Part model, mm, in its own coordinate system. Face numbers are marked on the shaded views. A direction names the side the tool comes from. Coordinates: 2 decimals unless noted, no trailing zeros. Write each loop counter-clockwise with the first axis right and the second up, starting at its lowest first coordinate (ties: lowest second). Pieces come first, ordered by that corner, then holes. Notation, with made-up numbers: (-12.5, -31.5) -> (19.5, -31.5) arc R24 cw to (19.5, -8.5) -> close; hole circle Ø6 at (-4.5, 76.25). An arc over 180 degrees is marked (long way). Write item = value, one per line. Start each with the question number.
Q1. Band-saw the part on C-C, the plane x = 29.5. List the corners of the cut face in (y, z).
Q2. Band-saw the part on D-D, the plane y = 8. List the corners of the cut face in (x, z).
Q3. Band-saw the part on A-A, the plane z = 28. List the corners of the cut face in (x, y).
Q4. Probe line 1 (Y direction, x = 29.5, z = 1.9); line 2 (Z direction, x = 1.65, y = 8); line 3 (Y direction, x = 14, z = 1). List the from-to ranges inside material, lowest first.
Q5. Band-saw the part on B-B, the plane y = 5. List the corners of the cut face in (x, z).
Q6. Pin check, flat tips, straight feed: P1, Ø6, axis at y = 13, z = 15, coming from the +X side; P2, Ø10, axis at x = 27.5, y = 3.5, coming from the +Z side. Stop position of each tip, or through.
Q7. Tool access for the marked faces 1 and 2: list every direction of +Z, -Z, +X, -X, +Y, -Y with a clear straight run to the whole face (end or side of a thin tool).
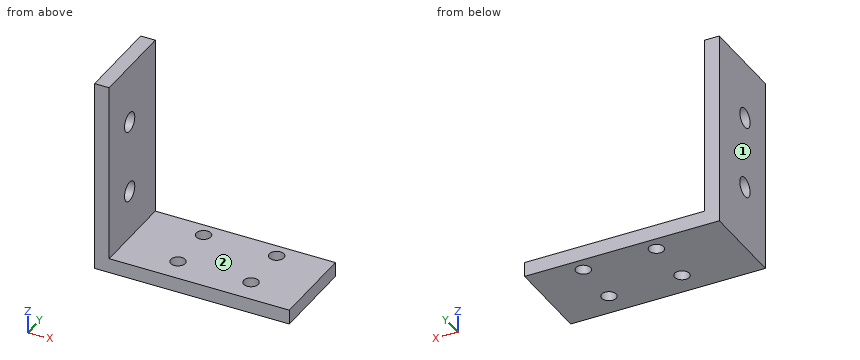
from build123d import *

# Parameters (mm, degrees)
ESQUISSE1_W             = 40
ESQUISSE1_H             = 18
BOSS_EXTRU_1_DEPTH      = 3
ESQUISSE2_W             = 3
ESQUISSE2_H             = 18
BOSS_EXTRU_2_DEPTH      = 37
ESQUISSE3_R             = 1.5
ENL_V_MAT_EXTRU_1_DEPTH = 58.384666942
ESQUISSE4_R             = 2
ENL_V_MAT_EXTRU_2_DEPTH = 58.384666942


with BuildPart() as part:
    # Esquisse1 → Boss.-Extru.1 (new body)
    with BuildSketch(Plane.XY):
        with Locations((20, 9)):
            Rectangle(ESQUISSE1_W, ESQUISSE1_H)
    extrude(amount=BOSS_EXTRU_1_DEPTH)

    # Esquisse2 → Boss.-Extru.2 (add)
    with BuildSketch(Plane.XY.offset(3)):
        with Locations((1.5, 9)):
            Rectangle(ESQUISSE2_W, ESQUISSE2_H)
    extrude(amount=BOSS_EXTRU_2_DEPTH)

    # Esquisse3 → Enlèv. mat.-Extru.1 (cut, through all)
    with BuildSketch(Plane.XY.offset(3)):
        with Locations((14.5, 15)):
            Circle(ESQUISSE3_R)
        with Locations((29.5, 15)):
            Circle(ESQUISSE3_R)
        with Locations((14.5, 5)):
            Circle(ESQUISSE3_R)
        with Locations((29.5, 5)):
            Circle(ESQUISSE3_R)
    extrude(amount=-ENL_V_MAT_EXTRU_1_DEPTH, mode=Mode.SUBTRACT)

    # Esquisse4 → Enlèv. mat.-Extru.2 (cut, through all)
    with BuildSketch(Plane(origin=(3, 0, 0), x_dir=(0, 0, -1), z_dir=(1, 0, 0))):
        with Locations(Location((-28, 8, 0), (0, 0, 90))):
            Circle(ESQUISSE4_R)
        with Locations(Location((-13, 8, 0), (0, 0, 90))):
            Circle(ESQUISSE4_R)
    extrude(amount=-ENL_V_MAT_EXTRU_2_DEPTH, mode=Mode.SUBTRACT)


solid = part.part
Ans:
q1.outline = (0, 0) -> (3.5, 0) -> (3.5, 3) -> (0, 3) -> close; (6.5, 0) -> (13.5, 0) -> (13.5, 3) -> (6.5, 3) -> close; (16.5, 0) -> (18, 0) -> (18, 3) -> (16.5, 3) -> close
q2.outline = (0, 0) -> (40, 0) -> (40, 3) -> (3, 3) -> (3, 11) -> (0, 11) -> close; (0, 15) -> (3, 15) -> (3, 26) -> (0, 26) -> close; (0, 30) -> (3, 30) -> (3, 40) -> (0, 40) -> close
q3.outline = (0, 0) -> (3, 0) -> (3, 6) -> (0, 6) -> close; (0, 10) -> (3, 10) -> (3, 18) -> (0, 18) -> close
q4.line_1 = 0 to 3.5, 6.5 to 13.5, 16.5 to 18
q4.line_2 = 0 to 11, 15 to 26, 30 to 40
q4.line_3 = 0 to 3.59, 6.41 to 13.59, 16.41 to 18
q5.outline = (0, 0) -> (13, 0) -> (13, 3) -> (3, 3) -> (3, 40) -> (0, 40) -> close; (16, 0) -> (28, 0) -> (28, 3) -> (16, 3) -> close; (31, 0) -> (40, 0) -> (40, 3) -> (31, 3) -> close
q6.P1 = 3
q6.P2 = 3
q7.face_1 = +Z, -Z, -X, +Y, -Y
q7.face_2 = +Z, +X, +Y, -Y
